Can you work these out from the model? Positions are in its coordinate system, mm. A direction names the side the tool comes from. Coordinates: 2 decimals unless noted, no trailing zeros. Order: outer loops, then holes, each group sorted by start corner. A loop starts at its lowest first (then second) coordinate and runs counter-clockwise, first axis right, second up. Notation, with made-up numbers: (-1, -4) -> (3, -4) arc R8 cw to (3, 1) -> close; hole circle Ø8 at (-24.75, 37). An arc over 180 degrees is marked (long way). Answer as a JSON object with one key per item and string values. Group by question number.
(1) Which directions (+Z, -Z, +X, -X, +Y, -Y) give clear straight access to the entire face, cutting with the end or side of a thin tool? Please do faces 1 (the flat face through (-0.5, 0, 3)), 2 (the flat face through (0.01, 8.43, 8.98)).
(2) If we mould it in two halves opening along Y, with no side actions, what happens to faces 3 (the cylindrical face through (-0.01, -15.93, 9.9)), 4 (the flat face through (0.007, -8.291, 8.937)), 5 (the flat face through (0.5, 0, 3))? For each: pulls with the +Y half, pulls with the -Y half, needs draft (parallel to the pull), parting line crosses it, or undercut.
(3) I want a section at A-A, the plane x = -0.1. List the corners of the cut face in (y, z) for me, plus the area to 3 significant figures.
(4) I need wall thicknesses on line 1 (Z direction, x = 0.05, y = 1.5); line 2 (Z direction, x = -0.1, y = -14.5); line 3 (Y direction, x = 0.25, z = -2.5). Which ranges of each line are inside material? Lowest first, please.
(5) I want a section at C-C, the plane z = -6.25. List the corners of the cut face in (x, y) for me.
(6) I want a section at B-B, the plane y = 0. List the corners of the cut face in (x, z) for me, plus the area to 3 significant figures.
Autodesk Inventor part; units mm, degrees
ref_plane "YZ Plane" through (0, 0, 0) normal (1, 0, 0) x (0, 1, 0)
ref_plane "XZ Plane" through (0, 0, 0) normal (0, 1, 0) x (-1, 0, 0)
ref_plane "XY Plane" through (0, 0, 0) normal (0, 0, 1) x (1, 0, 0)
sketch "スケッチ1" plane through (0, 0, 0) normal (0, 1, 0) x (-1, 0, 0)
  line L0 (-0.5, 7.5) -> (0.5, 7.5)
  line L1 (0.5, 7.5) -> (0.5, -7.5)
  line L2 (0.5, -7.5) -> (-0.5, -7.5)
  line L3 (-0.5, -7.5) -> (-0.5, 7.5)
  line L4 (-0.5, 7.5) -> (0.5, -7.5) construction
  line L5 (0.5, 7.5) -> (-0.5, -7.5) construction
  point P0 (0, 0)
  dimension "d0" = 1
  dimension "d1" = 15
extrude "押し出し1" add sketch "スケッチ1" along normal blind 3.5
sketch "スケッチ2" plane through (0.5, 0, 7.5) normal (1, 0, 0) x (0, 0, -1)
  line L0 (15, 3.5) -> (0, 3.5)
  line L1 (-3, 16.5) -> (0, 16.5)
  line L2 (0, 16.5) -> (15, 3.5)
  circle A0 centre (-1.5, 14.5) radius 0.25
  line L3 (-3, 16.5) -> (-3, 13.5)
  line L4 (-3, 13.5) -> (0, 3.5)
  point P0 (7.5, 0)
  point P1 (-1.5, 16.5)
  dimension "d5" = 3
  dimension "d6" = 0.5
  dimension "d7" = 2
  dimension "d11" = 13
  dimension "d12" = 3
  dimension "d13" = 3
extrude "押し出し2" add sketch "スケッチ2" against normal blind 1
fillet "フィレット1" radius 2 3 edges at (0, 16.5, 10.5) (0, 16.5, 7.5) (0, 13.5, 10.5)
mirror "ミラー1" about plane through (0, 0, 0) normal (0, -1, 0) of "押し出し2", "押し出し1", "フィレット1"
properties part number "TailHorn" material "ABS プラスチック"
Computed values:
{
 "1": {"face 1": "+Z, -Z, -X, +Y, -Y", "face 2": "+Z, +X, -X"},
 "2": {"face 3": "pulls with the -Y half", "face 4": "undercut", "face 5": "needs draft"},
 "3": {"outline": "(-16.5, 8.25) arc R2 ccw to (-16.01, 6.94) -> (-3.5, -7.5) -> (3.5, -7.5) -> (16.01, 6.94) arc R2 ccw to (16.5, 8.25) -> (16.5, 8.5) arc R2 ccw to (14.5, 10.5) -> (13.79, 10.5) arc R2 ccw to (13.22, 10.42) -> (3.5, 7.5) -> (-3.5, 7.5) -> (-13.22, 10.42) arc R2 ccw to (-13.79, 10.5) -> (-14.5, 10.5) arc R2 ccw to (-16.5, 8.5) -> close; hole circle Ø0.5 at (-14.5, 9); hole circle Ø0.5 at (14.5, 9)", "area": "346 mm2"},
 "4": {"line 1": "z = -7.5 to 7.5", "line 2": "z = 5.19 to 8.75, 9.25 to 10.5", "line 3": "y = -7.83 to 7.83"},
 "5": {"outline": "(-0.5, -4.58) -> (0.5, -4.58) -> (0.5, 4.58) -> (-0.5, 4.58) -> close"},
 "6": {"outline": "(-0.5, -7.5) -> (0.5, -7.5) -> (0.5, 7.5) -> (-0.5, 7.5) -> close", "area": "15.0 mm2"}
}
